Check sheet for the modelled part. Datum: model origin and axes. Units: mm. A direction names the side the tool comes from. Round coordinates to 2 decimals unless told otherwise and drop trailing zeros. Loops run counter-clockwise (first coordinate to the right, second up) from the corner with the lowest first, then second, coordinate; pieces in that order, holes last. Notation, with made-up numbers: (14.5, 71.5) - (71.5, 71.5) arc R23 ccw to (71.5, 103.5) - close; hole circle Ø7 at (20, -33.75). An arc over 180 degrees is marked (long way). Put each result on its own line as item: value. Start each with the question number.
Item 1: Section check C-C, the plane x = -3. Record the cut outline in (y, z).
Item 2: Tool access check on faces 4 (the flat face through (57.15, 0, 31)), 5 (the cylindrical face through (69.255, -31.736, 30.142)), 6 (the flat face through (70, 0, 12.7)). Record the directions out of +Z, -Z, +X, -X, +Y, -Y that give a thin tool (end or side, any length) a straight path to the whole face; none if there is none.
Item 3: Section check B-B, the plane z = 5. Record the cut outline in (x, y), and give its area (3 significant figures).
Item 4: Gauge pin test, flat ends, axial feed: pin 1 Ø6.5 at (x, y) = (69.85, 19.05) entering from -Z; pin 2 Ø8 at (y, z) = (8.5, 11.5) entering from -X; pin 3 Ø12 at (x, y) = (-11.5, -13.5) entering from -Z; pin 4 Ø2.5 at (y, z) = (-1, 30) entering from -X. Record the tip position at first contact, or that the pin passes through.
Item 5: Material ranges on line 1 along Y through (x, z) = (69, 19); line 2 along X through (y, z) = (9.5, -8); line 3 along Z through (x, y) = (-2, 19), recorded low to high.
Item 6: Section check D-D, the plane z = 14.5. Record the cut outline in (x, y), and give its area (3 significant figures).
Item 7: Draft check along X on faces 1 (the cylindrical face through (-15.12, 0.44, -11.59)), 2 (the cylindrical face through (68.884, 31.713, 30.142)), 3 (the cylindrical face through (32.197, -0.444, 8.881)). Enter one of: pulls with the +X half, pulls with the -X half, needs draft (parallel to the pull), parting line crosses it, or undercut.
Item 8: Section check A-A, the plane y = -1.5. Record the cut outline in (x, z) (3 decimals), and give its area (3 significant figures).
from build123d import *

# Parameters (mm, degrees)
F0_R     = 19.05
F1_DEPTH = 31.75
F3_DEPTH = 21.1074
F4_R     = 5.5626
F5_DEPTH = 62.3834


with BuildPart() as f1:
    # F0 (on Front) → F1 (new body, symmetric)
    with BuildSketch(Plane.XZ):
        with BuildLine():
            Line((69.85, 28.575), (0, 28.575))
            ThreePointArc((0, 28.575), (-20.205576, -20.205576), (28.575, 0))
            ThreePointArc((28.575, 0), (32.294744, 8.980256), (41.275, 12.7))
            Line((41.275, 12.7), (69.85, 12.7))
            Line((69.85, 12.7), (69.85, 28.575))
        make_face()
        Circle(F0_R, mode=Mode.SUBTRACT)
    extrude(amount=F1_DEPTH, both=True)

    # F2 (on face) → F3 (join)
    with BuildSketch(Plane(origin=(0, 0, 12.7), x_dir=(1, 0, 0), z_dir=(0, 0, -1))):
        with BuildLine():
            ThreePointArc((76.149155, 30.077721), (63.474628, 30.033835), (57.15, 19.05))
            Line((57.15, 19.05), (57.15, -19.05))
            ThreePointArc((57.15, -19.05), (63.474628, -30.033835), (76.149155, -30.077721))
            Line((76.149155, -30.077721), (109.499355, -11.027721))
            ThreePointArc((109.499355, -11.027721), (115.9002, 0), (109.499355, 11.027721))
            Line((109.499355, 11.027721), (76.149155, 30.077721))
        make_face()
    extrude(amount=-F3_DEPTH)

    # F4 (on face) → F5 (cut, through all)
    with BuildSketch(Plane.XY.offset(33.8074)):
        with Locations((103.2002, 0)):
            Circle(F4_R)
        with Locations((69.85, -19.05)):
            Circle(F4_R)
        with Locations((69.85, 19.05)):
            Circle(F4_R)
    extrude(amount=-F5_DEPTH, mode=Mode.SUBTRACT)


solid = f1.part
Check result:
1. outline: (-31.75, -28.42) - (31.75, -28.42) - (31.75, -18.81) - (-31.75, -18.81) - close; (-31.75, 18.81) - (31.75, 18.81) - (31.75, 28.42) - (-31.75, 28.42) - close
2. face 4: +Z, -X, +Y, -Y
2. face 5: +Z, -Y
2. face 6: -Z, +X, +Y, -Y
3. outline: (-28.13, -31.75) - (-18.38, -31.75) - (-18.38, 31.75) - (-28.13, 31.75) - close; (18.38, -31.75) - (29.6, -31.75) - (29.6, 31.75) - (18.38, 31.75) - close
3. area: 1,330 mm²
4. pin 1: through
4. pin 2: x = -27.57
4. pin 3: z = -28.04
4. pin 4: x = 57.15
5. line 1: -31.75 to -24.55, -13.55 to 13.55, 24.55 to 31.75
5. line 2: -27.43 to -17.29, 17.29 to 27.43
5. line 3: -28.5 to -18.94, 18.94 to 28.5
6. outline: (-24.62, -31.75) - (-12.36, -31.75) - (-12.36, 31.75) - (-24.62, 31.75) - close; (12.36, -31.75) - (69.85, -31.75) arc R12.7 ccw to (76.15, -30.08) - (109.5, -11.03) arc R12.7 ccw to (109.5, 11.03) - (76.15, 30.08) arc R12.7 ccw to (69.85, 31.75) - (12.36, 31.75) - close; hole circle Ø11.13 at (69.85, -19.05); hole circle Ø11.13 at (69.85, 19.05); hole circle Ø11.13 at (103.2, 0)
6. area: 6,000 mm²
7. face 1: undercut
7. face 2: parting line crosses it
7. face 3: pulls with the +X half
8. outline: (0, 28.575) arc R28.575 ccw (long way) to (28.575, 0) arc R12.7 cw to (41.275, 12.7) - (97.844, 12.7) - (97.844, 33.807) - (57.15, 33.807) - (57.15, 28.575) - close; (108.557, 12.7) - (115.811, 12.7) - (115.811, 33.807) - (108.557, 33.807) - close; hole circle Ø38.1 at (0, 0)
8. area: 3,100 mm²
